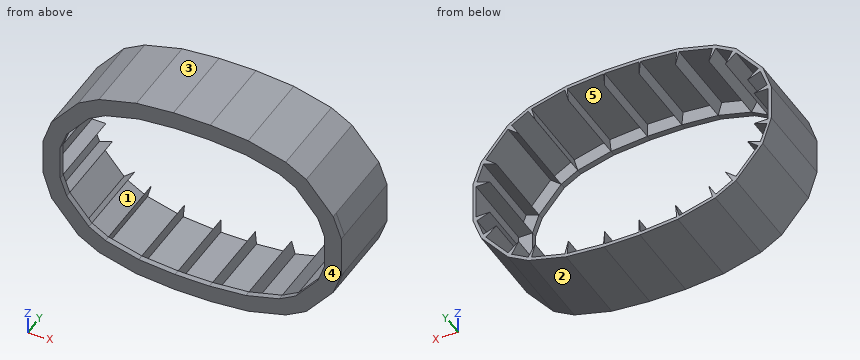
```python
from build123d import *

# Parameters (mm, degrees)
PAD_DEPTH          = 70
PAD001_DEPTH       = 5
PAD001_FACE43_W    = 70
PAD001_FACE43_H    = 30
POCKET_DEPTH       = 12
POCKET_FACE41_W    = 70
POCKET_FACE41_H    = 31.7305168913
POCKET001_DEPTH    = 12
POCKET001_FACE44_W = 70
POCKET001_FACE44_H = 30
POCKET002_DEPTH    = 12
POCKET002_FACE47_W = 70
POCKET002_FACE47_H = 31.7305168913
POCKET003_DEPTH    = 12
POCKET003_FACE37_W = 70
POCKET003_FACE37_H = 16.6623057169
POCKET004_DEPTH    = 12
POCKET004_FACE36_W = 70
POCKET004_FACE36_H = 30
POCKET005_DEPTH    = 12
POCKET005_FACE35_W = 70
POCKET005_FACE35_H = 16.6623057169
POCKET006_DEPTH    = 12
POCKET006_FACE34_W = 70
POCKET006_FACE34_H = 30
POCKET007_DEPTH    = 12
POCKET007_FACE33_W = 70
POCKET007_FACE33_H = 16.6623057169
POCKET008_DEPTH    = 12
POCKET008_FACE60_W = 70
POCKET008_FACE60_H = 30
POCKET009_DEPTH    = 12
POCKET009_FACE63_W = 70
POCKET009_FACE63_H = 16.6623057169
POCKET010_DEPTH    = 12
POCKET010_FACE66_W = 70
POCKET010_FACE66_H = 30
POCKET011_DEPTH    = 12
POCKET011_FACE69_W = 70
POCKET011_FACE69_H = 16.6623057169
POCKET012_DEPTH    = 12
POCKET012_FACE72_W = 70
POCKET012_FACE72_H = 30
POCKET013_DEPTH    = 12
POCKET013_FACE75_W = 70
POCKET013_FACE75_H = 16.6623057169
POCKET014_DEPTH    = 12
POCKET014_FACE78_W = 70
POCKET014_FACE78_H = 30
POCKET015_DEPTH    = 12
POCKET015_FACE81_W = 70
POCKET015_FACE81_H = 16.6623057169
POCKET016_DEPTH    = 12
POCKET016_FACE84_W = 70
POCKET016_FACE84_H = 30
POCKET017_DEPTH    = 12
POCKET017_FACE87_W = 70
POCKET017_FACE87_H = 31.7305168913
POCKET018_DEPTH    = 12
POCKET018_FACE32_W = 70
POCKET018_FACE32_H = 30
POCKET019_DEPTH    = 12
POCKET019_FACE31_W = 70
POCKET019_FACE31_H = 16.6623057169
POCKET020_DEPTH    = 12
POCKET020_FACE30_W = 70
POCKET020_FACE30_H = 30
POCKET021_DEPTH    = 12
POCKET021_FACE29_W = 70
POCKET021_FACE29_H = 31.7305168913
POCKET022_DEPTH    = 12
POCKET022_FACE98_W = 70
POCKET022_FACE98_H = 30
POCKET023_DEPTH    = 12


with BuildPart() as part:
    # Sketch → Pad (new body)
    with BuildSketch(Plane.XZ):
        Polygon((15.6005336184, 87.4879738248), (-16.433599, 87.4879738248), (-48.6209968735, 84.5990576256), (-81.2780534486, 75.8486256891), (-99.1915759479, 65.506248652), (-122.5813887031, 37.6313552709), (-129.9657652325, 16.0128529043), (-129.9657652325, -14.874853), (-122.5813887031, -37.6313552709), (-99.1915759479, -65.506248652), (-81.2780534486, -75.8486256891), (-48.6209968735, -84.5990576256), (-15.6005336184, -87.4879738248), (15.6005336184, -87.4879738248), (48.6209968735, -84.5990576256), (81.2780534486, -75.8486256891), (99.1915759479, -65.506248652), (122.5813887031, -37.6313552709), (129.6559912563, -18.1940445045), (129.6559912563, 18.1940445045), (122.5813887031, 37.6313552709), (99.1915759479, 65.506248652), (81.2780534486, 75.8486256891), (48.6209968735, 84.5990576256), align=None)
        Polygon((-115, 15), (-115, -15), (-109.3011558106, -30.6574457275), (-90.01752752, -53.638779021), (-75.5875474835, -61.9699318795), (-46.6097726948, -69.7345032326), (-15, -72.5), (15, -72.5), (46.6097726948, -69.7345032326), (75.5875474835, -61.9699318795), (90.01752752, -53.638779021), (109.3011558106, -30.6574457275), (115, -15), (115, 15), (109.3011558106, 30.6574457275), (90.01752752, 53.638779021), (75.5875474835, 61.9699318795), (46.6097726948, 69.7345032326), (15, 72.5), (-15, 72.5), (-46.6097726948, 69.7345032326), (-75.5875474835, 61.9699318795), (-90.01752752, 53.638779021), (-109.3011558106, 30.6574457275), align=None, mode=Mode.SUBTRACT)
    extrude(amount=PAD_DEPTH)

    # Pad Face50 → Pad001 (add)
    with BuildSketch(Plane(origin=(0.0330089745, -70, 0.0202146999), x_dir=(-1, 0, 0), z_dir=(0, -1, 0))):
        Polygon((-15.5675246439, -87.4677591249), (16.4666079745, -87.4677591249), (48.654005848, -84.5788429257), (81.3110624231, -75.8284109892), (99.2245849224, -65.4860339521), (122.6143976776, -37.611140571), (129.998774207, -15.9926382044), (129.998774207, 14.8950676999), (122.6143976776, 37.6515699708), (99.2245849224, 65.5264633519), (81.3110624231, 75.868840389), (48.654005848, 84.6192723255), (15.633542593, 87.5081885247), (-15.5675246439, 87.5081885247), (-48.5879878989, 84.6192723255), (-81.2450444741, 75.868840389), (-99.1585669734, 65.5264633519), (-122.5483797286, 37.6515699708), (-129.6229822817, 18.2142592044), (-129.6229822817, -18.1738298046), (-122.5483797286, -37.611140571), (-99.1585669734, -65.4860339521), (-81.2450444741, -75.8284109892), (-48.5879878989, -84.5788429257), align=None)
        Polygon((15.0330089745, -72.4797853001), (-14.9669910255, -72.4797853001), (-46.5767637203, -69.7142885327), (-75.554538509, -61.9497171796), (-89.9845185454, -53.6185643211), (-109.268146836, -30.6372310276), (-114.9669910255, -14.9797853001), (-114.9669910255, 15.0202146999), (-109.268146836, 30.6776604274), (-89.9845185454, 53.6589937209), (-75.554538509, 61.9901465794), (-46.5767637203, 69.7547179325), (-14.9669910255, 72.5202146999), (15.0330089745, 72.5202146999), (46.6427816693, 69.7547179325), (75.620556458, 61.9901465794), (90.0505364945, 53.6589937209), (109.3341647851, 30.6776604274), (115.0330089745, 15.0202146999), (115.0330089745, -14.9797853001), (109.3341647851, -30.6372310276), (90.0505364945, -53.6185643211), (75.620556458, -61.9497171796), (46.6427816693, -69.7142885327), align=None, mode=Mode.SUBTRACT)
    extrude(amount=PAD001_DEPTH)

    # Pad001 Face43 → Pocket (cut)
    with BuildSketch(Plane(origin=(-61.0986600892, -35, -65.852217556), x_dir=(0, 1, 0), z_dir=(0.2588190451, 0, 0.9659258263))):
        Rectangle(PAD001_FACE43_W, PAD001_FACE43_H)
    extrude(amount=-POCKET_DEPTH, mode=Mode.SUBTRACT)

    # Pocket Face41 → Pocket001 (cut)
    with BuildSketch(Plane(origin=(-30.8048863474, -35, -71.1172516163), x_dir=(0, 1, 0), z_dir=(0.0871557427, 0, 0.9961946981))):
        Rectangle(POCKET_FACE41_W, POCKET_FACE41_H)
    extrude(amount=-POCKET001_DEPTH, mode=Mode.SUBTRACT)

    # Pocket001 Face44 → Pocket002 (cut)
    with BuildSketch(Plane(origin=(0, -35, -72.5), x_dir=(0, 1, 0), z_dir=(0, 0, 1))):
        Rectangle(POCKET001_FACE44_W, POCKET001_FACE44_H)
    extrude(amount=-POCKET002_DEPTH, mode=Mode.SUBTRACT)

    # Pocket002 Face47 → Pocket003 (cut)
    with BuildSketch(Plane(origin=(30.8048863474, -35, -71.1172516163), x_dir=(0, 1, 0), z_dir=(-0.0871557427, 0, 0.9961946981))):
        Rectangle(POCKET002_FACE47_W, POCKET002_FACE47_H)
    extrude(amount=-POCKET003_DEPTH, mode=Mode.SUBTRACT)

    # Pocket003 Face37 → Pocket004 (cut)
    with BuildSketch(Plane(origin=(-82.8025375017, -35, -57.8043554503), x_dir=(0, -1, 0), z_dir=(0.5, 0, 0.8660254038))):
        Rectangle(POCKET003_FACE37_W, POCKET003_FACE37_H)
    extrude(amount=-POCKET004_DEPTH, mode=Mode.SUBTRACT)

    # Pocket004 Face36 → Pocket005 (cut)
    with BuildSketch(Plane(origin=(-99.6593416653, -35, -42.1481123743), x_dir=(0, -1, 0), z_dir=(0.7660444431, 0, 0.6427876097))):
        Rectangle(POCKET004_FACE36_W, POCKET004_FACE36_H)
    extrude(amount=-POCKET005_DEPTH, mode=Mode.SUBTRACT)

    # Pocket005 Face35 → Pocket006 (cut)
    with BuildSketch(Plane(origin=(-112.1505779053, -35, -22.8287228637), x_dir=(0, -1, 0), z_dir=(0.9396926208, 0, 0.3420201433))):
        Rectangle(POCKET005_FACE35_W, POCKET005_FACE35_H)
    extrude(amount=-POCKET006_DEPTH, mode=Mode.SUBTRACT)

    # Pocket006 Face34 → Pocket007 (cut)
    with BuildSketch(Plane(origin=(-115, -35, 0), x_dir=(0, -1, 0), z_dir=(1, 0, 0))):
        Rectangle(POCKET006_FACE34_W, POCKET006_FACE34_H)
    extrude(amount=-POCKET007_DEPTH, mode=Mode.SUBTRACT)

    # Pocket007 Face33 → Pocket008 (cut)
    with BuildSketch(Plane(origin=(-112.1505779053, -35, 22.8287228637), x_dir=(0, -1, 0), z_dir=(0.9396926208, 0, -0.3420201433))):
        Rectangle(POCKET007_FACE33_W, POCKET007_FACE33_H)
    extrude(amount=-POCKET008_DEPTH, mode=Mode.SUBTRACT)

    # Pocket008 Face60 → Pocket009 (cut)
    with BuildSketch(Plane(origin=(61.0986600892, -35, -65.852217556), x_dir=(0, 1, 0), z_dir=(-0.2588190451, 0, 0.9659258263))):
        Rectangle(POCKET008_FACE60_W, POCKET008_FACE60_H)
    extrude(amount=-POCKET009_DEPTH, mode=Mode.SUBTRACT)

    # Pocket009 Face63 → Pocket010 (cut)
    with BuildSketch(Plane(origin=(82.8025375017, -35, -57.8043554503), x_dir=(0, 1, 0), z_dir=(-0.5, 0, 0.8660254038))):
        Rectangle(POCKET009_FACE63_W, POCKET009_FACE63_H)
    extrude(amount=-POCKET010_DEPTH, mode=Mode.SUBTRACT)

    # Pocket010 Face66 → Pocket011 (cut)
    with BuildSketch(Plane(origin=(99.6593416653, -35, -42.1481123743), x_dir=(0, 1, 0), z_dir=(-0.7660444431, 0, 0.6427876097))):
        Rectangle(POCKET010_FACE66_W, POCKET010_FACE66_H)
    extrude(amount=-POCKET011_DEPTH, mode=Mode.SUBTRACT)

    # Pocket011 Face69 → Pocket012 (cut)
    with BuildSketch(Plane(origin=(112.1505779053, -35, -22.8287228637), x_dir=(0, 1, 0), z_dir=(-0.9396926208, 0, 0.3420201433))):
        Rectangle(POCKET011_FACE69_W, POCKET011_FACE69_H)
    extrude(amount=-POCKET012_DEPTH, mode=Mode.SUBTRACT)

    # Pocket012 Face72 → Pocket013 (cut)
    with BuildSketch(Plane(origin=(115, -35, 0), x_dir=(0, 1, 0), z_dir=(-1, 0, 0))):
        Rectangle(POCKET012_FACE72_W, POCKET012_FACE72_H)
    extrude(amount=-POCKET013_DEPTH, mode=Mode.SUBTRACT)

    # Pocket013 Face75 → Pocket014 (cut)
    with BuildSketch(Plane(origin=(112.1505779053, -35, 22.8287228637), x_dir=(0, 1, 0), z_dir=(-0.9396926208, 0, -0.3420201433))):
        Rectangle(POCKET013_FACE75_W, POCKET013_FACE75_H)
    extrude(amount=-POCKET014_DEPTH, mode=Mode.SUBTRACT)

    # Pocket014 Face78 → Pocket015 (cut)
    with BuildSketch(Plane(origin=(99.6593416653, -35, 42.1481123743), x_dir=(0, 1, 0), z_dir=(-0.7660444431, 0, -0.6427876097))):
        Rectangle(POCKET014_FACE78_W, POCKET014_FACE78_H)
    extrude(amount=-POCKET015_DEPTH, mode=Mode.SUBTRACT)

    # Pocket015 Face81 → Pocket016 (cut)
    with BuildSketch(Plane(origin=(82.8025375017, -35, 57.8043554503), x_dir=(0, 1, 0), z_dir=(-0.5, 0, -0.8660254038))):
        Rectangle(POCKET015_FACE81_W, POCKET015_FACE81_H)
    extrude(amount=-POCKET016_DEPTH, mode=Mode.SUBTRACT)

    # Pocket016 Face84 → Pocket017 (cut)
    with BuildSketch(Plane(origin=(61.0986600892, -35, 65.852217556), x_dir=(0, -1, 0), z_dir=(-0.2588190451, 0, -0.9659258263))):
        Rectangle(POCKET016_FACE84_W, POCKET016_FACE84_H)
    extrude(amount=-POCKET017_DEPTH, mode=Mode.SUBTRACT)

    # Pocket017 Face87 → Pocket018 (cut)
    with BuildSketch(Plane(origin=(30.8048863474, -35, 71.1172516163), x_dir=(0, -1, 0), z_dir=(-0.0871557427, 0, -0.9961946981))):
        Rectangle(POCKET017_FACE87_W, POCKET017_FACE87_H)
    extrude(amount=-POCKET018_DEPTH, mode=Mode.SUBTRACT)

    # Pocket018 Face32 → Pocket019 (cut)
    with BuildSketch(Plane(origin=(-99.6593416653, -35, 42.1481123743), x_dir=(0, -1, 0), z_dir=(0.7660444431, 0, -0.6427876097))):
        Rectangle(POCKET018_FACE32_W, POCKET018_FACE32_H)
    extrude(amount=-POCKET019_DEPTH, mode=Mode.SUBTRACT)

    # Pocket019 Face31 → Pocket020 (cut)
    with BuildSketch(Plane(origin=(-82.8025375017, -35, 57.8043554503), x_dir=(0, -1, 0), z_dir=(0.5, 0, -0.8660254038))):
        Rectangle(POCKET019_FACE31_W, POCKET019_FACE31_H)
    extrude(amount=-POCKET020_DEPTH, mode=Mode.SUBTRACT)

    # Pocket020 Face30 → Pocket021 (cut)
    with BuildSketch(Plane(origin=(-61.0986600892, -35, 65.852217556), x_dir=(0, -1, 0), z_dir=(0.2588190451, 0, -0.9659258263))):
        Rectangle(POCKET020_FACE30_W, POCKET020_FACE30_H)
    extrude(amount=-POCKET021_DEPTH, mode=Mode.SUBTRACT)

    # Pocket021 Face29 → Pocket022 (cut)
    with BuildSketch(Plane(origin=(-30.8048863474, -35, 71.1172516163), x_dir=(0, -1, 0), z_dir=(0.0871557427, 0, -0.9961946981))):
        Rectangle(POCKET021_FACE29_W, POCKET021_FACE29_H)
    extrude(amount=-POCKET022_DEPTH, mode=Mode.SUBTRACT)

    # Pocket022 Face98 → Pocket023 (cut)
    with BuildSketch(Plane(origin=(0, -35, 72.5), x_dir=(0, -1, 0), z_dir=(0, 0, -1))):
        Rectangle(POCKET022_FACE98_W, POCKET022_FACE98_H)
    extrude(amount=-POCKET023_DEPTH, mode=Mode.SUBTRACT)


solid = part.part
```
Input: part model. Units: mm. Frame: model coordinates. Face numbers are marked on the shaded views. A direction names the side the tool comes from. Give positions to 0.01 mm unless a question says otherwise; leave off trailing zeros. Order: outer loops, then holes, each group sorted by start corner. A loop starts at its lowest first (then second) coordinate and runs counter-clockwise, first axis right, second up. Notation, with made-up numbers: (43, 10) - (51, 10) arc R18 ccw to (51, 39) - close; hole circle Ø1 at (69, -15). An arc over 180 degrees is marked (long way). One line per item, written item: value.
1. Cut plane B-B, the plane x = -23. Output: boundary loops of the cut face in (y, z), and give its area (3 significant figures).
Determined:
outline: (-75, -86.84) - (0, -86.84) - (0, -83.85) - (-70, -83.85) - (-70, -71.8) - (-75, -71.8) - close; (-75, 71.8) - (-70, 71.8) - (-70, 83.85) - (0, 83.85) - (0, 86.9) - (-75, 86.9) - close
area: 574 mm2
2. Pin query (flat end, axial travel): pin 1 Ø12 at (x, y) = (-70.5, -52.5) entering from -Z; pin 2 Ø5 at (x, z) = (-84, -63.5) entering from +Y; pin 3 Ø1 at (y, z) = (-15.5, -25) entering from -X. Return the tip coordinate at first contact, or that it passes through.
Determined:
pin 1: z = -80.34
pin 2: y = -70
pin 3: x = -126.84
3. Cut plane A-A, the plane z = -4.5. Output: boundary loops of the cut face in (x, y).
Determined:
outline: (-129.97, -75) - (-115, -75) - (-115, -70) - (-127, -70) - (-127, 0) - (-129.97, 0) - close; (115, -75) - (129.66, -75) - (129.66, 0) - (127, 0) - (127, -70) - (115, -70) - close
4. Reachability of the marked faces 4 and 5 from +Z, -Z, +X, -X, +Y, -Y: full face, straight path, thin tool, end or side. Return the list, or none.
Determined:
face 4: +Z, -Z, +X, -X, -Y
face 5: +Y
5. Line query: probe 1 along Z at (x, y) = (-2, -19); probe 2 along X at (y, z) = (-9, -68.5); probe 3 along X at (y, z) = (-66, -61). Output: solid intervals per line, ascending.
Determined:
probe 1: -87.49 to -84.5, 84.5 to 87.49
probe 2: -94.01 to -88.28, -79.36 to -77.34, 77.34 to 79.36, 88.28 to 94.01
probe 3: -102.97 to -99.51, -98.79 to -94.27, 94.27 to 98.79, 99.51 to 102.97
6. Draft query along X for the marked faces 1, 2 and 3. Return one class per face: released by +X, released by -X, zero draft, split by the parting line, or undercut.
Determined:
face 1: undercut
face 2: released by +X
face 3: released by -X
